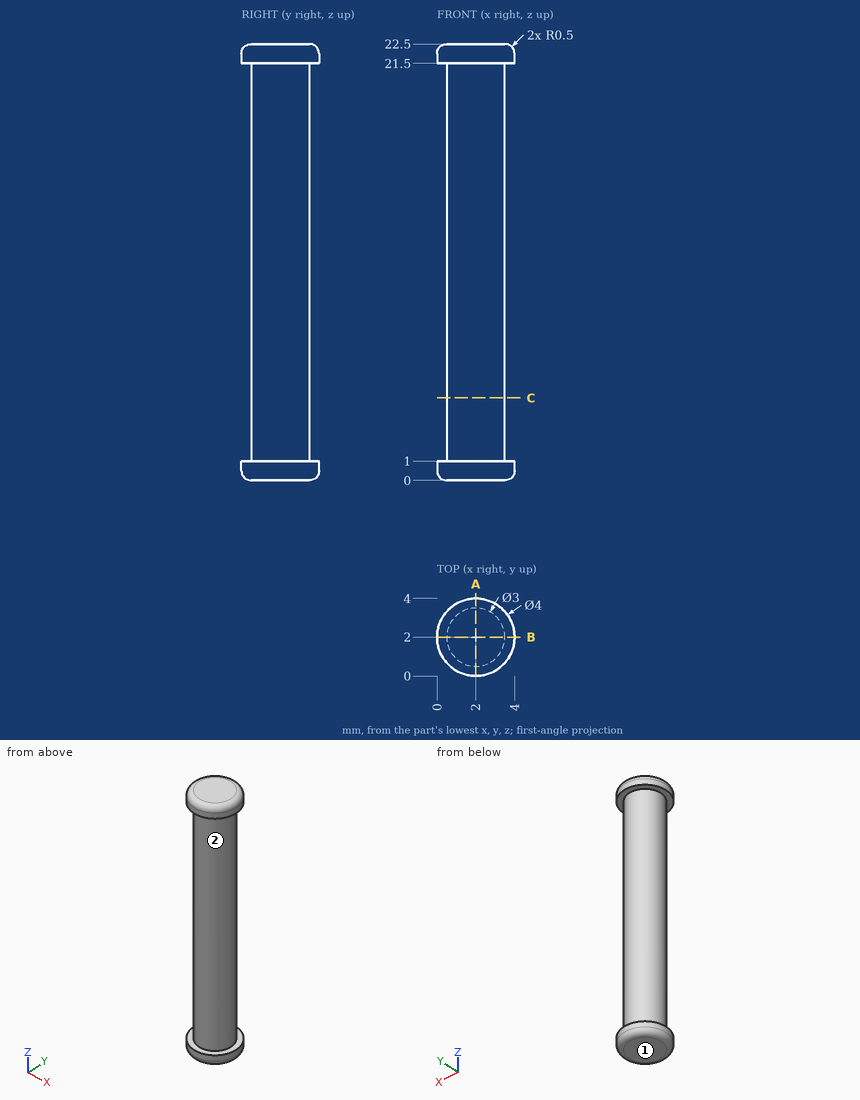
Part print with two shaded views. Sizes in mm from the minimum x, y, z corner. A direction names the side the tool comes from. Give positions to 0.01 mm unless a question says otherwise; leave off trailing zeros. Order: outer loops, then holes, each group sorted by start corner. A loop starts at its lowest first (then second) coordinate and runs counter-clockwise, first axis right, second up. Notation, with made-up numbers: M 53,32 L 91,32 A20 ccw 91,68 Z; hole C 71,-10 d9. An arc over 180 degrees is marked long. Put each result on its own line as item: value.
Item 1: Drop a flat-ended pin along its axis: pin 1 Ø2 at (x, z) = (2.5, 16) entering from +Y. Give the stop position or say it passes through.
Results are:
pin 1: y = 3.5
Item 2: Which spindle directions (+Z, -Z, +X, -X, +Y, -Y) get a long thin tool onto all of the face, cutting with end or side? Do the marked faces 1 and 2. Say none if no direction does.
Results are:
face 1: -Z, +X, -X, +Y, -Y
face 2: none
Item 3: Cut at A-A on x = 2. Write the cut outline in (y, z), then the cut area to 3 significant figures.
Results are:
outline: M 0,0.5 A0.5 ccw 0.5,0 L 3.5,0 A0.5 ccw 4,0.5 L 4,1 L 3.5,1 L 3.5,21.5 L 4,21.5 L 4,22 A0.5 ccw 3.5,22.5 L 0.5,22.5 A0.5 ccw 0,22 L 0,21.5 L 0.5,21.5 L 0.5,1 L 0,1 Z
area: 69.3 mm2
Item 4: Cut at C-C on z = 4.25. Write the cut outline in (x, y), then the cut area to 3 significant figures.
Results are:
outline: C 2,2 d3
area: 7.07 mm2
Item 5: Wall check: probe 1 along Z at (x, y) = (2.4, 0.4); probe 2 along Z at (x, y) = (0.7, 0.55); probe 3 along Y at (x, z) = (3.3, 13.75). Give the ranges that are in metal, low to high.
Results are:
probe 1: 0.02 to 1, 21.5 to 22.48
probe 2: 0.28 to 1, 21.5 to 22.22
probe 3: 1.25 to 2.75
